Geometry check sheet. Reference: drawing and pictorial views, mm from the part's lowest x, y, z. A direction names the side the tool comes from. Round coordinates to 2 decimals unless told otherwise and drop trailing zeros. Order: outer loops, then holes, each group sorted by start corner. A loop starts at its lowest first (then second) coordinate and runs counter-clockwise, first axis right, second up.
(1) Cross-section at D-D on z = 22. Enter the section's corners in (x, y), and give its area (3 significant figures).
(2) Cross-section at A-A on z = 9.5. Enter the section's corners in (x, y).
(3) Cross-section at C-C on x = 12.5. Enter the section's corners in (y, z).
(4) Gauge pin test, flat ends, axial feed: P1, Ø1, axis at x = 10.5, y = 3, coming from the -Z side; P2, Ø1, axis at x = 10.5, y = 3.5, coming from the +Z side; P3, Ø1, axis at y = 2, z = 8, coming from the +X side. Record the tip position at first contact, or that the pin passes through.
(5) Cross-section at B-B on x = 23. Enter the section's corners in (y, z).
(6) Set-up check for the marked faces 1, 2 and 3: record each of +Z, -Z, +X, -X, +Y, -Y from which the full face is reachable in a straight line by a thin tool's end or side.
(7) Thickness scan on L1, parallel to X at y = 0.65, z = 22; L2, parallel to Z at x = 23, y = 0.5; L3, parallel to X at y = 3.5, z = 10.5. Record the ranges inside material, lowest first.
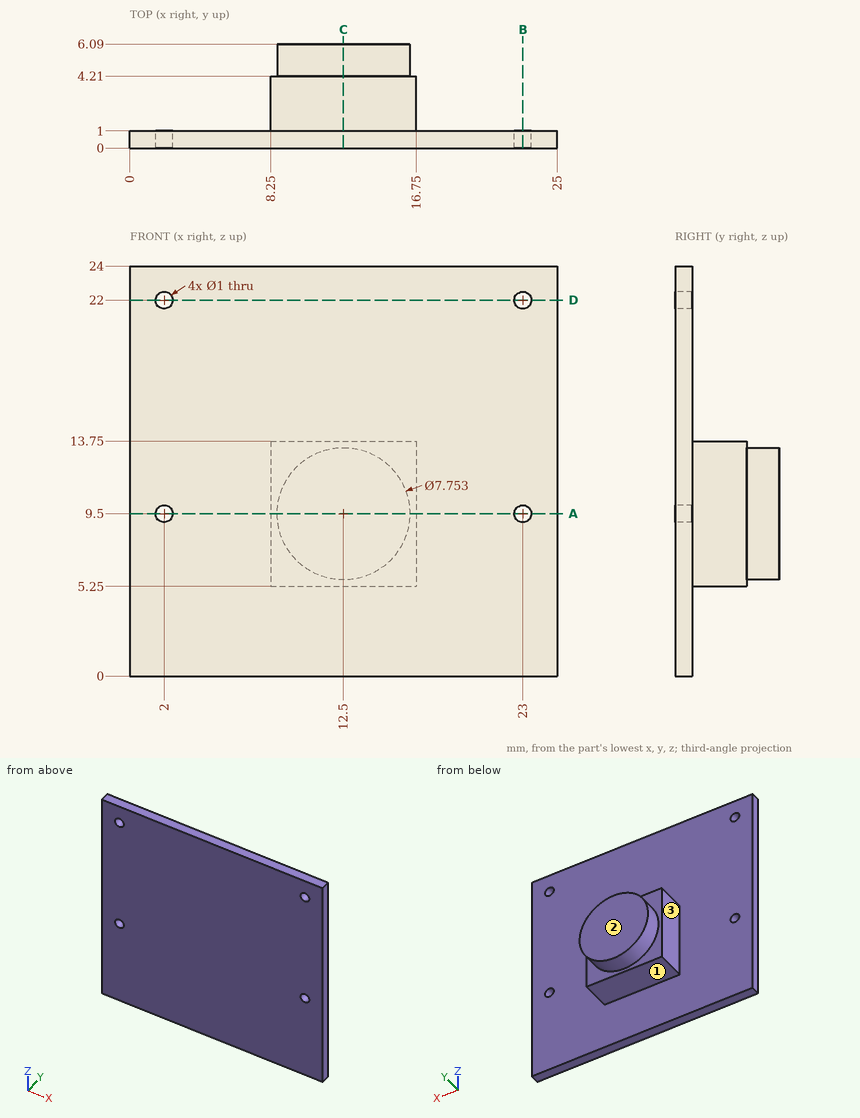
Found:
1. outline: (0, 0) - (1.5, 0) - (1.5, 1) - (0, 1) - close; (2.5, 0) - (22.5, 0) - (22.5, 1) - (2.5, 1) - close; (23.5, 0) - (25, 0) - (25, 1) - (23.5, 1) - close
1. area: 23.0 mm2
2. outline: (0, 0) - (1.5, 0) - (1.5, 1) - (0, 1) - close; (2.5, 0) - (22.5, 0) - (22.5, 1) - (16.75, 1) - (16.75, 4.21) - (16.38, 4.21) - (16.38, 6.09) - (8.62, 6.09) - (8.62, 4.21) - (8.25, 4.21) - (8.25, 1) - (2.5, 1) - close; (23.5, 0) - (25, 0) - (25, 1) - (23.5, 1) - close
3. outline: (0, 0) - (1, 0) - (1, 5.25) - (4.21, 5.25) - (4.21, 5.62) - (6.09, 5.62) - (6.09, 13.38) - (4.21, 13.38) - (4.21, 13.75) - (1, 13.75) - (1, 24) - (0, 24) - close
4. P1: stops at z = 5.25
4. P2: stops at z = 13.75
4. P3: stops at x = 16.75
5. outline: (0, 0) - (1, 0) - (1, 9) - (0, 9) - close; (0, 10) - (1, 10) - (1, 21.5) - (0, 21.5) - close; (0, 22.5) - (1, 22.5) - (1, 24) - (0, 24) - close
6. face 1: -Z, +X, -X, +Y
6. face 2: +Z, -Z, +X, -X, +Y
6. face 3: +Z, -Z, -X, +Y
7. L1: x = 0 to 1.5, 2.5 to 22.5, 23.5 to 25
7. L2: z = 0 to 9, 10 to 21.5, 22.5 to 24
7. L3: x = 8.25 to 16.75
